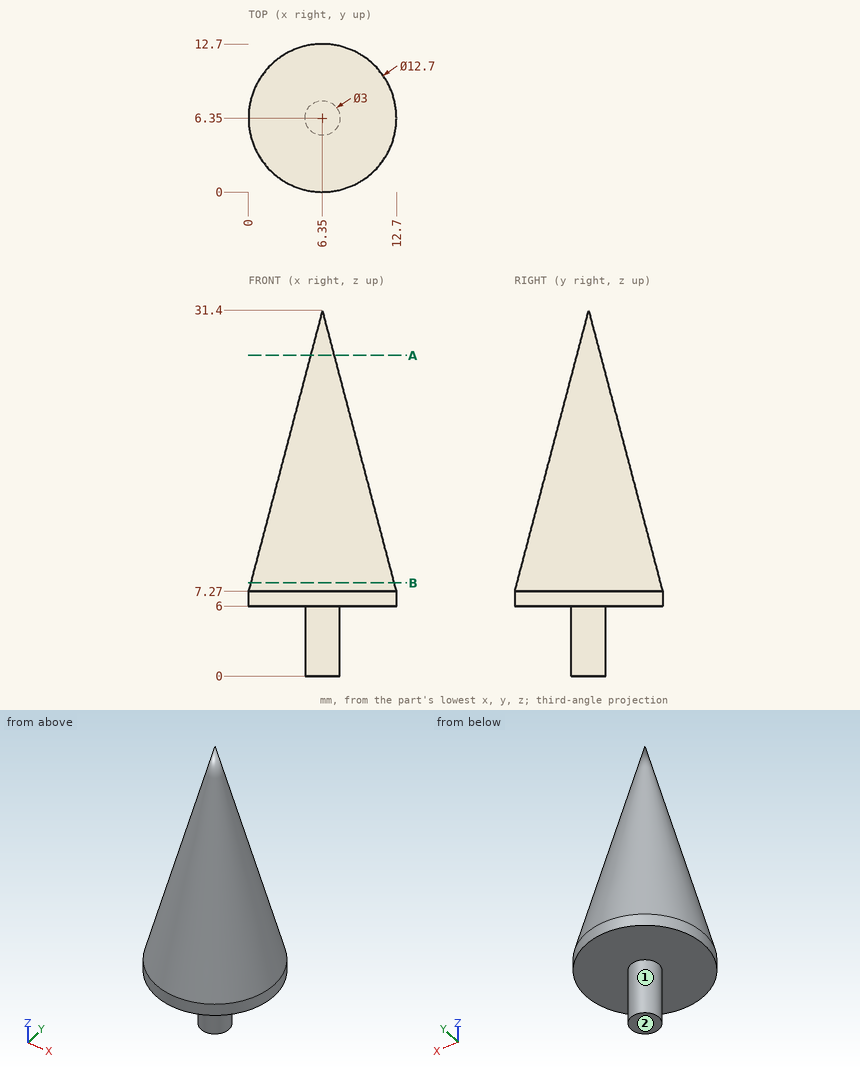
Verification items for this drawing (mm, ordinates from the low corner). A direction names the side the tool comes from. Coordinates: 2 decimals unless noted, no trailing zeros. Write each loop counter-clockwise with the first axis right and the second up, starting at its lowest first coordinate (ties: lowest second). Pieces come first, ordered by that corner, then holes. Notation, with made-up numbers: M -13,-7 L 28,-7 A7 cw 28,5 Z; hole C -12,50 d9. An arc over 180 degrees is marked long. Use one line per item in the form item = value. Start each with the question number.
1) Section check A-A on z = 27.5. Enter the section's corners in (x, y).
2) Section check B-B on z = 8. Enter the section's corners in (x, y), and give its area (3 significant figures).
3) Thickness scan on probe 1 along X at (y, z) = (6.25, 26); probe 2 along Y at (x, z) = (3, 16.5); probe 3 along X at (y, z) = (2.75, 16). Record the ranges inside material, lowest first. Write a range as from..to.
4) Go/stop test with flat-tipped pins: pin 1 Ø4 at (x, z) = (11, 20) entering from -Y; pin 2 Ø2 at (y, z) = (7.5, 7.5) entering from +X; pin 3 Ø4 at (y, z) = (6, 22) entering from -X. Record where each tip stops, or that it passes through.
5) Set-up check for the marked faces 1 and 2: record each of +Z, -Z, +X, -X, +Y, -Y from which the full face is reachable in a straight line by a thin tool's end or side.
Responses:
q1.outline = C 6.35,6.35 d2.05
q2.outline = C 6.35,6.35 d12.32
q2.area = 119 mm2
q3.probe_1 = 4.93..7.77
q3.probe_2 = 4.31..8.39
q3.probe_3 = 4.49..8.21
q4.pin_1 = 4.78
q4.pin_2 = 12.7
q4.pin_3 = 3.36
q5.face_1 = -Z
q5.face_2 = -Z, +X, -X, +Y, -Y
